```python
from build123d import *

# Parameters (mm, degrees)
F0_W = 13
F0_H = 5
F2_R = 2
F3_R = 0.5


with BuildPart() as f1:
    # F0 (on Front) → F1 (revolve)
    with BuildSketch(Plane.XZ):
        with Locations((6.5, 2.5)):
            Rectangle(F0_W, F0_H)
        Polygon((13, 5), (13, 0), (14.236494, 0), align=None)
    revolve(axis=Axis((0, 0, 2.5), (0, 0, 1)))

    # F2
    f2_edges = [f1.edges().sort_by_distance(p)[0] for p in [
        (-13, 0, 5),
    ]]
    fillet(f2_edges, radius=F2_R)

    # F3
    f3_edges = [f1.edges().sort_by_distance(p)[0] for p in [
        (-14.236494, 0, 0),
    ]]
    fillet(f3_edges, radius=F3_R)


solid = f1.part
```
Can you work these out from the model? Positions are in its coordinate system, mm. Round coordinates to 2 decimals unless told otherwise and drop trailing zeros. Loops run counter-clockwise (first coordinate to the right, second up) from the corner with the lowest first, then second, coordinate; pieces in that order, holes last. Notation, with made-up numbers: (27.5, 43) -> (56.5, 43) arc R23 cw to (56.5, 66) -> close; hole circle Ø4 at (-32.5, -16.5). An arc over 180 degrees is marked (long way). One line per item, written item: value. Start each with the question number.
1. If we section it at C-C, the plane z = 4.55: Write out the boundary of the cut face in (x, y), then the cut area to 3 significant figures.
2. For pin 1 (3 mm diameter, centred on y = 1.5, z = 1.5, fed in from +X); pin 2 (2 mm diameter, centred on y = 2.5, z = 0.5, fed in from -X), each with a flat end and sliding along its axis, tell me the tip position at first contact or that it passes through.
3. If we section it at A-A, the plane y = 0: Write out the boundary of the cut face in (x, z), then the cut area to 3 significant figures.
4. If I drill on probe 1 along X at (y, z) = (-5, 3.4); probe 2 along X at (y, z) = (7.5, 2.9); probe 3 along Y at (x, z) = (-3.75, 2.75), over which ranges is the centre line in solid material (lowest first)?
Calculated:
1. outline: circle Ø25.4 at (0, 0)
1. area: 507 mm²
2. pin 1: stops at x = 14.09
2. pin 2: stops at x = -14.02
3. outline: (-14.08, 0.62) arc R0.5 ccw to (-13.6, 0) -> (13.6, 0) arc R0.5 ccw to (14.08, 0.62) -> (13.38, 3.48) arc R2 ccw to (11.43, 5) -> (-11.43, 5) arc R2 ccw to (-13.38, 3.48) -> close
3. area: 135 mm²
4. probe 1: x = -12.43 to 12.43
4. probe 2: x = -11.25 to 11.25
4. probe 3: y = -13.03 to 13.03
